from build123d import *

# Parameters (mm, degrees)
F0_R     = 5.5
F0_R_2   = 12
F1_DEPTH = 4


with BuildPart() as f1:
    # F0 (on Top) → F1 (new body)
    with BuildSketch(Plane.XY):
        Polygon((50, 50), (0, 50), (-50, 50), (-50, -70), (0, -70), (50, -70), align=None)
        with Locations((-34, -54)):
            Circle(F0_R, mode=Mode.SUBTRACT)
        with Locations((34, -54)):
            Circle(F0_R, mode=Mode.SUBTRACT)
        with Locations((0, -35)):
            Circle(F0_R, mode=Mode.SUBTRACT)
        with Locations((-34, 0)):
            Circle(F0_R, mode=Mode.SUBTRACT)
        Circle(F0_R_2, mode=Mode.SUBTRACT)
        with Locations((34, 0)):
            Circle(F0_R, mode=Mode.SUBTRACT)
    extrude(amount=F1_DEPTH)


solid = f1.part
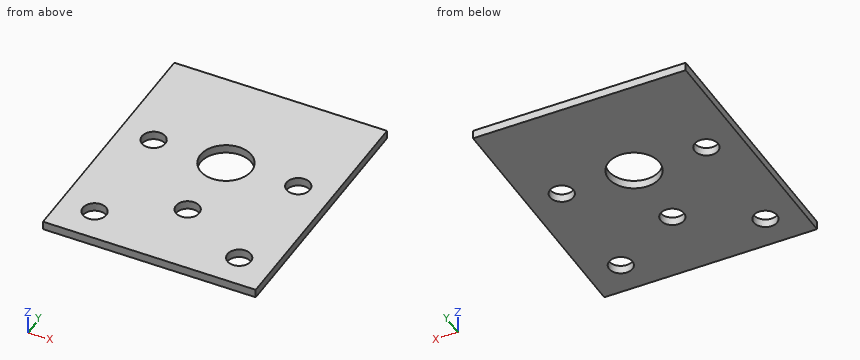
The listing builds one solid part. Answer for the finished solid, in the listing's coordinates (mm). Give positions to 0.01 mm unless a question says otherwise; leave off trailing zeros. Loops run counter-clockwise (first coordinate to the right, second up) from the corner with the lowest first, then second, coordinate; pieces in that order, holes last.
Item 1: A cutting plane is placed at D-D (y = 0). Give the vertices of the cut face in (x, z), then the cut area to 3 significant figures.
Derived:
outline: (-50, 0) - (-39.5, 0) - (-39.5, 4) - (-50, 4) - close; (-28.5, 0) - (-12, 0) - (-12, 4) - (-28.5, 4) - close; (12, 0) - (28.5, 0) - (28.5, 4) - (12, 4) - close; (39.5, 0) - (50, 0) - (50, 4) - (39.5, 4) - close
area: 216 mm2
Item 2: Find the intervals of material crossed by line 1 along Y through (x, z) = (34, 2.85); line 2 along Y through (x, z) = (-32, 2.5); line 3 along X through (y, z) = (-58.5, 3), in increasing order.
Derived:
line 1: y = -70 to -59.5, -48.5 to -5.5, 5.5 to 50
line 2: y = -70 to -59.12, -48.88 to -5.12, 5.12 to 50
line 3: x = -50 to -37.16, -30.84 to 30.84, 37.16 to 50
Item 3: A cutting plane is placed at A-A (y = -35). Give the vertices of the cut face in (x, z), then the cut area to 3 significant figures.
Derived:
outline: (-50, 0) - (-5.5, 0) - (-5.5, 4) - (-50, 4) - close; (5.5, 0) - (50, 0) - (50, 4) - (5.5, 4) - close
area: 356 mm2
Item 4: A cutting plane is placed at B-B (x = 34). Give the vertices of the cut face in (y, z), then the cut area to 3 significant figures.
Derived:
outline: (-70, 0) - (-59.5, 0) - (-59.5, 4) - (-70, 4) - close; (-48.5, 0) - (-5.5, 0) - (-5.5, 4) - (-48.5, 4) - close; (5.5, 0) - (50, 0) - (50, 4) - (5.5, 4) - close
area: 392 mm2
Item 5: A cutting plane is placed at C-C (z = 2.85). Give the vertices of the cut face in (x, y).
Derived:
outline: (-50, -70) - (50, -70) - (50, 50) - (-50, 50) - close; hole circle Ø11 at (-34, -54); hole circle Ø11 at (-34, 0); hole circle Ø24 at (0, 0); hole circle Ø11 at (0, -35); hole circle Ø11 at (34, -54); hole circle Ø11 at (34, 0)
